Design review of the part shown in the three views and the two pictorial views. Dimensions are in mm from the part's minimum x, y and z. A direction names the side the tool comes from. Round coordinates to 2 decimals unless told otherwise and drop trailing zeros. Loops run counter-clockwise (first coordinate to the right, second up) from the corner with the lowest first, then second, coordinate; pieces in that order, holes last. Notation, with made-up numbers: M -31.5,50 L -15.5,50 A14 ccw -15.5,76 Z; hole C 55.5,37.5 d9. An arc over 180 degrees is marked long. Return JSON: item names as keys, results as strings. Group by question number.
Q1. Clearance check with flat-ended pins moving along their axes: pin 1 Ø5.5 at (y, z) = (7.5, 8) entering from +X; pin 2 Ø3 at (x, z) = (12.5, 4.5) entering from -Y; pin 3 Ø2 at (x, z) = (21, 5) entering from +Y. State where each tip first meets the part, or that it passes through.
Q2. Consider section B-B (y = 3.5). State the section outline as (x, z) points, and give its area (3 significant figures).
Q3. Consider section C-C (x = 20.2). State the section outline as (y, z) points.
Q4. For the marked faces 4, 5, 6, 7 and 8, list the 3-axis set-ups (+Z, -Z, +X, -X, +Y, -Y) from which the entire face can be reached by the end or side of a thin tool; tool diameter is ignored.
Q5. To check wall thickness, follow line 1 along X through (y, z) = (1.9, 4.2); line 2 along X through (y, z) = (3.75, 0.5); line 3 along X through (y, z) = (2.5, 9.75). State the ranges of each line that lie inside material, in increasing order.
Q6. Draft analysis for pull direction X (two halves, no side actions). For the marked faces 1, 2 and 3, state which applies: pulls with the +X half, pulls with the -X half, needs draft (parallel to the pull), parting line crosses it, or undercut.
Q7. Consider section D-D (z = 7.25). State the section outline as (x, y) points, and give its area (3 significant figures).
Q8. Consider section A-A (z = 4.2). State the section outline as (x, y) points, and give its area (3 significant figures).
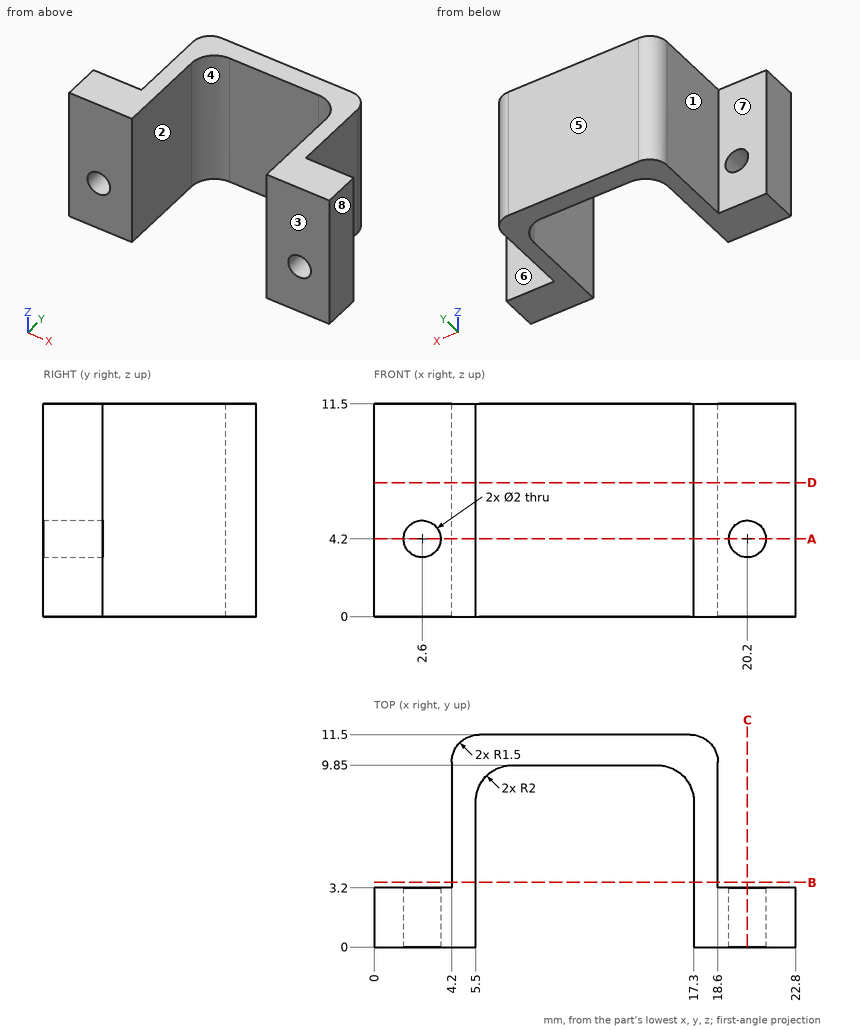
Values:
{
 "1": {"pin 1": "stops at x = 18.6", "pin 2": "stops at y = 9.85", "pin 3": "stops at y = 3.2"},
 "2": {"outline": "M 4.2,0 L 5.5,0 L 5.5,11.5 L 4.2,11.5 Z; M 17.3,0 L 18.6,0 L 18.6,11.5 L 17.3,11.5 Z", "area": "29.9 mm2"},
 "3": {"outline": "M 0,0 L 3.2,0 L 3.2,3.2 L 0,3.2 Z; M 0,5.2 L 3.2,5.2 L 3.2,11.5 L 0,11.5 Z"},
 "4": {"face 4": "+Z, -Z, -Y", "face 5": "+Z, -Z, +X, -X, +Y", "face 6": "+Z, -Z, +X, +Y", "face 7": "+Z, -Z, -X, +Y", "face 8": "+Z, -Z, +X, +Y, -Y"},
 "5": {"line 1": "x = 0 to 1.6, 3.6 to 5.5, 17.3 to 19.2, 21.2 to 22.8", "line 2": "x = 4.2 to 5.5, 17.3 to 18.6", "line 3": "x = 0 to 5.5, 17.3 to 22.8"},
 "6": {"face 1": "pulls with the -X half", "face 2": "undercut", "face 3": "needs draft"},
 "7": {"outline": "M 0,0 L 5.5,0 L 5.5,7.85 A2 cw 7.5,9.85 L 15.3,9.85 A2 cw 17.3,7.85 L 17.3,0 L 22.8,0 L 22.8,3.2 L 18.6,3.2 L 18.6,10 A1.5 ccw 17.1,11.5 L 5.7,11.5 A1.5 ccw 4.2,10 L 4.2,3.2 L 0,3.2 Z", "area": "77.0 mm2"},
 "8": {"outline": "M 0,0 L 1.6,0 L 1.6,3.2 L 0,3.2 Z; M 3.6,0 L 5.5,0 L 5.5,7.85 A2 cw 7.5,9.85 L 15.3,9.85 A2 cw 17.3,7.85 L 17.3,0 L 19.2,0 L 19.2,3.2 L 18.6,3.2 L 18.6,10 A1.5 ccw 17.1,11.5 L 5.7,11.5 A1.5 ccw 4.2,10 L 4.2,3.2 L 3.6,3.2 Z; M 21.2,0 L 22.8,0 L 22.8,3.2 L 21.2,3.2 Z", "area": "64.2 mm2"}
}
